from build123d import *

# Parameters (mm, degrees)
SKETCH1_W           = 45.956077194
SKETCH1_H           = 60.759300765
BOSS_EXTRUDE1_DEPTH = 4.800000052
SKETCH2_W           = 36.889410711
SKETCH2_H           = 52.292642565
CUT_EXTRUDE1_DEPTH  = 105.99289819
SKETCH3_W           = 9.066666483
SKETCH3_H           = 43.825967432
CUT_EXTRUDE3_DEPTH  = 105.99289819
SKETCH4_W           = 29.02274386
SKETCH4_H           = 8.4666582
CUT_EXTRUDE4_DEPTH  = 90.963914511


with BuildPart() as part:
    # Sketch1 → Boss-Extrude1 (new body)
    with BuildSketch(Plane(origin=(0, 0, 0), x_dir=(1, 0, 0), z_dir=(0, 1, 0))):
        with Locations((-66.116726553, -24.961035308)):
            Rectangle(SKETCH1_W, SKETCH1_H)
    extrude(amount=BOSS_EXTRUDE1_DEPTH)

    # Sketch2 → Cut-Extrude1 (cut, through all)
    with BuildSketch(Plane(origin=(0, 4.800000052, 0), x_dir=(1, 0, 0), z_dir=(0, 1, 0))):
        with Locations((-70.650059795, -29.194364408)):
            Rectangle(SKETCH2_W, SKETCH2_H)
    extrude(amount=-CUT_EXTRUDE1_DEPTH, mode=Mode.SUBTRACT)

    # Sketch3 → Cut-Extrude3 (cut, through all)
    with BuildSketch(Plane(origin=(0, 4.800000052, 0), x_dir=(1, 0, 0), z_dir=(0, 1, 0))):
        with Locations((-47.672021198, -33.427701974)):
            Rectangle(SKETCH3_W, SKETCH3_H)
    extrude(amount=-CUT_EXTRUDE3_DEPTH, mode=Mode.SUBTRACT)

    # Sketch4 → Cut-Extrude4 (cut, through all)
    with BuildSketch(Plane(origin=(0, 4.800000052, 0), x_dir=(1, 0, 0), z_dir=(0, 1, 0))):
        with Locations((-74.58339322, 1.185285975)):
            Rectangle(SKETCH4_W, SKETCH4_H)
    extrude(amount=-CUT_EXTRUDE4_DEPTH, mode=Mode.SUBTRACT)


solid = part.part
Work out the finished part from the listing and answer in its coordinate system (mm). A direction names the side the tool comes from. Coordinates: 2 decimals unless noted, no trailing zeros. Write each loop counter-clockwise with the first axis right and the second up, starting at its lowest first coordinate (ties: lowest second). Pieces come first, ordered by that corner, then holes.
1. The part is cut by section B-B, the plane x = -59. Write down the section's boundary in (y, z).
Results list:
outline: (0, -5.42) - (4.8, -5.42) - (4.8, 3.05) - (0, 3.05) - close
2. For faces 1 (the flat face through (-50, 0, 1)), 2 (the flat face through (-52.205, 2, 7)), determine the directions among +Z, -Z, +X, -X, +Y, -Y from which every point of the face is accessible in a straight line to the end or side of a thin tool.
Results list:
face 1: +Z, -Z, +X, -X, -Y
face 2: +Z, -X, +Y, -Y
3. A flat-ended cylindrical pin translates along its axis: pin 1 (1.5 mm diameter, centred on x = -55, y = 0.5, fed in from +Z). Find the tip coordinate at first contact, or state that the pin passes through.
Results list:
pin 1: stops at z = 3.05
4. The part is cut by section C-C, the plane z = 5.5. Write down the section's boundary in (x, y).
Results list:
outline: (-52.21, 0) - (-43.14, 0) - (-43.14, 4.8) - (-52.21, 4.8) - close
5. The part is cut by section A-A, the plane y = 2. Write down the section's boundary in (x, z).
Results list:
outline: (-60.07, -5.42) - (-43.14, -5.42) - (-43.14, 11.51) - (-52.21, 11.51) - (-52.21, 3.05) - (-60.07, 3.05) - close
6. Consider line 1 along X through (y, z) = (2.1, 7.75); line 2 along Z through (x, y) = (-54.75, 0.95). Determine where each line is inside the solid, lowest interval first.
Results list:
line 1: x = -52.21 to -43.14
line 2: z = -5.42 to 3.05
